Source: CAD feature listing. Evaluate the final solid. Frame: model axes, mm. Face numbers are marked on the shaded views. A direction names the side the tool comes from. Coordinates: 2 decimals unless noted, no trailing zeros. Write each loop counter-clockwise with the first axis right and the second up, starting at its lowest first coordinate (ties: lowest second). Pieces come first, ordered by that corner, then holes. Notation, with made-up numbers: (25.25, 29) - (71.25, 29) arc R10 ccw to (71.25, 35) - close; hole circle Ø4 at (85.25, 9). An arc over 180 degrees is marked (long way). One line per item, written item: value.
from build123d import *

# Parameters (mm, degrees)
SKETCH2_W           = 10
SKETCH2_H           = 30
SKETCH2_R           = 2.5
BOSS_EXTRUDE1_DEPTH = 5
SKETCH3_W           = 30
SKETCH3_H           = 30
BOSS_EXTRUDE2_DEPTH = 2
SKETCH4_W           = 2
SKETCH4_H           = 30
BOSS_EXTRUDE3_DEPTH = 20
SKETCH5_W           = 30
SKETCH5_H           = 50
BOSS_EXTRUDE4_DEPTH = 18.5
CUT_EXTRUDE1_DEPTH  = 15
BOSS_EXTRUDE5_DEPTH = 5
SKETCH9_W           = 30
SKETCH9_H           = 50
CUT_EXTRUDE2_DEPTH  = 3
CUT_EXTRUDE3_DEPTH  = 10
FILLET1_R           = 5
SKETCH13_W          = 2.5
SKETCH13_H          = 30
CUT_EXTRUDE4_DEPTH  = 8
BOSS_EXTRUDE9_DEPTH = 5
SKETCH15_W          = 30
SKETCH15_H          = 1
CUT_EXTRUDE5_DEPTH  = 1
CUT_EXTRUDE6_DEPTH  = 50.117206761


with BuildPart() as part:
    # Sketch2 → Boss-Extrude1 (new body)
    with BuildSketch(Plane.XY):
        Rectangle(SKETCH2_W, SKETCH2_H)
        with Locations((0, 10)):
            Circle(SKETCH2_R, mode=Mode.SUBTRACT)
        with Locations((0, -10)):
            Circle(SKETCH2_R, mode=Mode.SUBTRACT)
    extrude(amount=BOSS_EXTRUDE1_DEPTH)

    # Sketch3 → Boss-Extrude2 (add)
    with BuildSketch(Plane(origin=(5, 0, 0), x_dir=(0, 0, -1), z_dir=(1, 0, 0))):
        with Locations((-2.5, 0)):
            Rectangle(SKETCH3_W, SKETCH3_H)
    extrude(amount=BOSS_EXTRUDE2_DEPTH)

    # Sketch4 → Boss-Extrude3 (add)
    with BuildSketch(Plane.XZ.offset(15)):
        with Locations((6, 2.5)):
            Rectangle(SKETCH4_W, SKETCH4_H)
    extrude(amount=BOSS_EXTRUDE3_DEPTH)

    # Sketch5 → Boss-Extrude4 (add)
    with BuildSketch(Plane(origin=(7, 0, 0), x_dir=(0, 0, -1), z_dir=(1, 0, 0))):
        with Locations((-2.5, -10)):
            Rectangle(SKETCH5_W, SKETCH5_H)
    extrude(amount=BOSS_EXTRUDE4_DEPTH)

    # Sketch6 → Cut-Extrude1 (cut)
    with BuildSketch(Plane.ZY.offset(-5)):
        Polygon((-12.5, 15), (-12.5, -35), (17.5, -35), (17.5, 15), (5, 15), (5, -15), (0, -15), (0, 15), align=None)
    extrude(amount=-CUT_EXTRUDE1_DEPTH, mode=Mode.SUBTRACT)

    # Sketch7 → Boss-Extrude5 (add)
    with BuildSketch(Plane.XY):
        Polygon((-5, -15), (20, -35), (20, -15), align=None)
    extrude(amount=BOSS_EXTRUDE5_DEPTH)

    # Sketch9 → Cut-Extrude2 (cut)
    with BuildSketch(Plane(origin=(25.5, 0, 0), x_dir=(0, 0, -1), z_dir=(1, 0, 0))):
        with Locations((-2.5, -10)):
            Rectangle(SKETCH9_W, SKETCH9_H)
    extrude(amount=-CUT_EXTRUDE2_DEPTH, mode=Mode.SUBTRACT)

    # Sketch12 → Cut-Extrude3 (cut)
    with BuildSketch(Plane.XY.offset(5)):
        Polygon((2.123696111, 15), (20, 0), (20, 15), align=None)
    extrude(amount=-CUT_EXTRUDE3_DEPTH, mode=Mode.SUBTRACT)

    # Fillet1
    fillet1_edges = [part.edges().sort_by_distance(p)[0] for p in [
        (2.123696111, 15, 2.5),
        (-5, -15, 2.5),
        (-5, 15, 2.5),
    ]]
    fillet(fillet1_edges, radius=FILLET1_R)

    # Sketch13 → Cut-Extrude4 (cut)
    with BuildSketch(Plane(origin=(0, 15, 0), x_dir=(1, 0, 0), z_dir=(0, 1, 0))):
        with Locations((21.25, -2.5)):
            Rectangle(SKETCH13_W, SKETCH13_H)
    extrude(amount=-CUT_EXTRUDE4_DEPTH, mode=Mode.SUBTRACT)

    # Sketch14 → Boss-Extrude9 (add)
    with BuildSketch(Plane.XZ.offset(35)):
        Polygon((22.5, -12.5), (22.5, 17.5), (20, 17.5), (20, 5), (20, 0), (20, -12.5), align=None)
    extrude(amount=BOSS_EXTRUDE9_DEPTH)

    # Sketch15 → Cut-Extrude5 (cut)
    with BuildSketch(Plane(origin=(22.5, 0, 0), x_dir=(0, 0, -1), z_dir=(1, 0, 0))):
        with Locations((-2.5, 4.5)):
            Rectangle(SKETCH15_W, SKETCH15_H)
        with Locations((-2.5, 1.5)):
            Rectangle(SKETCH15_W, SKETCH15_H)
        with Locations((-2.5, -1.5)):
            Rectangle(SKETCH15_W, SKETCH15_H)
        with Locations((-2.5, -4.5)):
            Rectangle(SKETCH15_W, SKETCH15_H)
        with Locations((-2.5, -7.5)):
            Rectangle(SKETCH15_W, SKETCH15_H)
        with Locations((-2.5, -10.5)):
            Rectangle(SKETCH15_W, SKETCH15_H)
        with Locations((-2.5, -13.5)):
            Rectangle(SKETCH15_W, SKETCH15_H)
        with Locations((-2.5, -16.5)):
            Rectangle(SKETCH15_W, SKETCH15_H)
        with Locations((-2.5, -19.5)):
            Rectangle(SKETCH15_W, SKETCH15_H)
        with Locations((-2.5, -22.5)):
            Rectangle(SKETCH15_W, SKETCH15_H)
        with Locations((-2.5, -25.5)):
            Rectangle(SKETCH15_W, SKETCH15_H)
        with Locations((-2.5, -28.5)):
            Rectangle(SKETCH15_W, SKETCH15_H)
        with Locations((-2.5, -31.5)):
            Rectangle(SKETCH15_W, SKETCH15_H)
        with Locations((-2.5, -34.5)):
            Rectangle(SKETCH15_W, SKETCH15_H)
        with Locations((-2.5, -37.5)):
            Rectangle(SKETCH15_W, SKETCH15_H)
    extrude(amount=-CUT_EXTRUDE5_DEPTH, mode=Mode.SUBTRACT)

    # Sketch17 → Cut-Extrude6 (cut, through all)
    with BuildSketch(Plane.XY.offset(5)):
        Polygon((8, -0.374062741), (8, -15.15500122), (16, -21.55500122), (16, -7.08685979), align=None)
    extrude(amount=-CUT_EXTRUDE6_DEPTH, mode=Mode.SUBTRACT)


solid = part.part
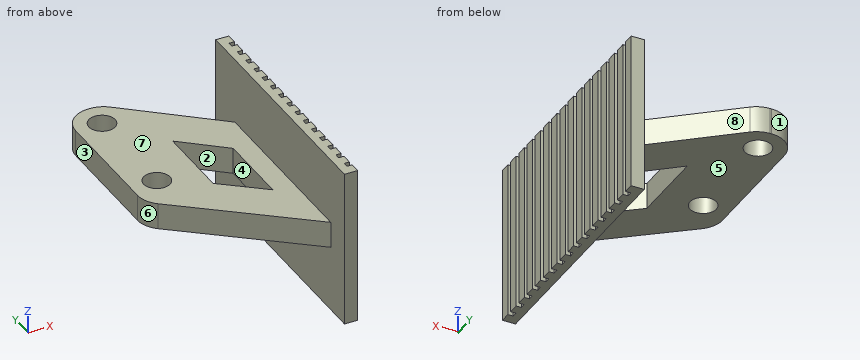
1) Section query C-C on y = -30. Output: boundary loops of the cut face in (x, z).
Values found:
outline: (13.75, 0) - (20, 0) - (20, -12.5) - (22.5, -12.5) - (22.5, 17.5) - (20, 17.5) - (20, 5) - (13.75, 5) - close
2) Draft query along Y for the marked faces 1, 2 and 3. Return one class per face: released by +Y, released by -Y, zero draft, split by the parting line, or undercut.
Values found:
face 1: released by +Y
face 2: undercut
face 3: zero draft
3) Section query D-D on x = 1.5. Output: boundary loops of the cut face in (y, z), then the cut area to 3 significant figures.
Values found:
outline: (-20.2, 0) - (-12, 0) - (-12, 5) - (-20.2, 5) - close; (-8, 0) - (8, 0) - (8, 5) - (-8, 5) - close; (12, 0) - (14.85, 0) - (14.85, 5) - (12, 5) - close
area: 135 mm2
4) Material intervals for line 1 (Y direction, x = 0, z = 3.85); line 2 (Z direction, x = 4.75, y = 2); line 3 (X direction, y = -28.5, z = 9.5), sorted ascending.
Values found:
line 1: -19 to -12.5, -7.5 to 7.5, 12.5 to 15
line 2: 0 to 5
line 3: 20 to 21.5
5) Reachability of the marked faces 4, 5, 6, 7 and 8 from +Z, -Z, +X, -X, +Y, -Y: full face, straight path, thin tool, end or side. Return the list, or none.
Values found:
face 4: +Z, -Z
face 5: -Z, -X, +Y, -Y
face 6: +Z, -Z, -X, -Y
face 7: +Z, -X, +Y, -Y
face 8: +Z, -Z, +Y
6) Section query A-A on x = 10. Output: boundary loops of the cut face in (y, z) (3 decimals), then the cut area to 3 significant figures.
Values found:
outline: (-27, 0) - (-16.755, 0) - (-16.755, 5) - (-27, 5) - close; (-2.052, 0) - (8.391, 0) - (8.391, 5) - (-2.052, 5) - close
area: 103 mm2
7) Contact query for flat-ended pins moving along their axis: P1, Ø0.5, axis at y = -1.5, z = 5.5, coming from the +X side; P2, Ø1, axis at y = -33, z = 1, coming from the -X side (3 decimals); P3, Ø1.5, axis at x = 11, y = -4.5, coming from the -Z side; P4, Ø8, axis at y = -12.5, z = -4.5, coming from the -X side. Output: stop coordinate, or through.
Values found:
P1: x = 21.5
P2: x = 16.875
P3: through
P4: x = 20
8) Section query B-B on y = 11. Output: boundary loops of the cut face in (x, z).
Values found:
outline: (-4.9, 0) - (-2.29, 0) - (-2.29, 5) - (-4.9, 5) - close; (2.29, 0) - (6.89, 0) - (6.89, 5) - (2.29, 5) - close
